```python
from build123d import *

# Parameters (mm, degrees)
F0_W     = 10
F0_H     = 5
F0_W_2   = 5
F0_H_2   = 10
F1_DEPTH = 5
F2_R     = 2.5
F3_DEPTH = 5


with BuildPart() as f1:
    # F0 (on Top) → F1 (new body)
    with BuildSketch(Plane.XY):
        Polygon((-5, 25), (-40, 25), (-40, 5), (-40, -5), (-40, -25), (-5, -25), (5, -25), (40, -25), (40, -5), (40, 5), (40, 25), (5, 25), align=None)
        with Locations((0, 27.5)):
            Rectangle(F0_W, F0_H)
        with Locations((-42.5, 0)):
            Rectangle(F0_W_2, F0_H_2)
        with Locations((0, -27.5)):
            Rectangle(F0_W, F0_H)
        with Locations((42.5, 0)):
            Rectangle(F0_W_2, F0_H_2)
    extrude(amount=F1_DEPTH)

    # F2 (on face) → F3 (cut)
    with BuildSketch(Plane.XY.offset(5)):
        with Locations((-27, 10)):
            Circle(F2_R)
        with Locations((-14, 10)):
            Circle(F2_R)
        with Locations((0, 10)):
            Circle(F2_R)
        with Locations((14, 10)):
            Circle(F2_R)
        with Locations((27, 10)):
            Circle(F2_R)
        with Locations((-27, 0)):
            Circle(F2_R)
        with Locations((-14, 0)):
            Circle(F2_R)
        Circle(F2_R)
        with Locations((14, 0)):
            Circle(F2_R)
        with Locations((27, 0)):
            Circle(F2_R)
        with Locations((27, -10)):
            Circle(F2_R)
        with Locations((14, -10)):
            Circle(F2_R)
        with Locations((0, -10)):
            Circle(F2_R)
        with Locations((-14, -10)):
            Circle(F2_R)
        with Locations((-27, -10)):
            Circle(F2_R)
    extrude(amount=-F3_DEPTH, mode=Mode.SUBTRACT)


solid = f1.part
```
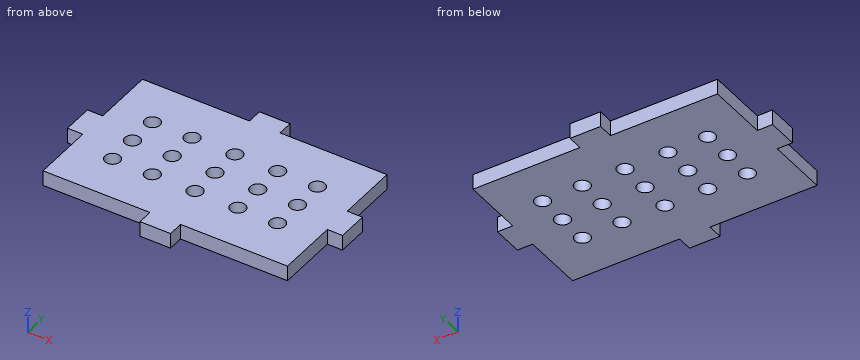
Could you check a few things on this model? Use its own coordinates, in mm. Round coordinates to 2 decimals unless told otherwise and drop trailing zeros. Write each loop counter-clockwise with the first axis right and the second up, starting at its lowest first coordinate (ties: lowest second). Pieces come first, ordered by that corner, then holes. Notation, with made-up numbers: M 75,76.25 L 82,76.25 A25 cw 82,102.25 Z; hole C 33,-3 d8. An arc over 180 degrees is marked long. Answer in a Markdown table with one row per item. Add a question column.
Q1. Will these pins go through, and if not, where does the flat tip stop? pin 1 Ø1 at (x, y) = (12, 13) entering from -Z; pin 2 Ø2.5 at (x, z) = (17.5, 3.5) entering from +Y; pin 3 Ø2.5 at (y, z) = (-12, 3) entering from +X.
Q2. Imagine slicing it at C-C (y = 1.5). Please give me the cut outline in (x, z), then the cut area to 3 significant figures.
Q3. Imagine slicing it at D-D (z = 3.45). Give the number of separate pieces and of enclosed holes in the cut face, then the cut area to 3 significant figures.
Q4. Imagine slicing it at A-A (y = -10). Please give me the cut outline in (x, z).
Q5. Imagine slicing it at B-B (x = 14). Please give me the cut outline in (y, z), then the cut area to 3 significant figures.
Q6. If I drill on line 1 (Y direction, x = 27, z = 2.05); line 2 (Y direction, x = 0, z = 2.35); line 3 (X direction, y = 13.5, z = 1.75), over which ranges is the centre line in solid material (lowest first)? Write a range as from..to.
Values:
| question | item | result |
|---|---|---|
| 1 | pin 1 | z = 0 |
| 1 | pin 2 | y = 25 |
| 1 | pin 3 | x = 40 |
| 2 | outline | M -45,0 L -29,0 L -29,5 L -45,5 Z; M -25,0 L -16,0 L -16,5 L -25,5 Z; M -12,0 L -2,0 L -2,5 L -12,5 Z; M 2,0 L 12,0 L 12,5 L 2,5 Z; M 16,0 L 25,0 L 25,5 L 16,5 Z; M 29,0 L 45,0 L 45,5 L 29,5 Z |
| 2 | area | 350 mm^2 |
| 3 | separate pieces | 1 |
| 3 | enclosed holes | 15 |
| 3 | area | 3,910 mm^2 |
| 4 | outline | M -40,0 L -29.5,0 L -29.5,5 L -40,5 Z; M -24.5,0 L -16.5,0 L -16.5,5 L -24.5,5 Z; M -11.5,0 L -2.5,0 L -2.5,5 L -11.5,5 Z; M 2.5,0 L 11.5,0 L 11.5,5 L 2.5,5 Z; M 16.5,0 L 24.5,0 L 24.5,5 L 16.5,5 Z; M 29.5,0 L 40,0 L 40,5 L 29.5,5 Z |
| 5 | outline | M -25,0 L -12.5,0 L -12.5,5 L -25,5 Z; M -7.5,0 L -2.5,0 L -2.5,5 L -7.5,5 Z; M 2.5,0 L 7.5,0 L 7.5,5 L 2.5,5 Z; M 12.5,0 L 25,0 L 25,5 L 12.5,5 Z |
| 5 | area | 175 mm^2 |
| 6 | line 1 | -25..-12.5, -7.5..-2.5, 2.5..7.5, 12.5..25 |
| 6 | line 2 | -30..-12.5, -7.5..-2.5, 2.5..7.5, 12.5..30 |
| 6 | line 3 | -40..40 |
